Geometry: see drawing. Coordinates: mm, zero at the bounding-box minimum. Round coordinates to 2 decimals unless told otherwise and drop trailing zeros. Order: outer loops, then holes, each group sorted by start corner. A loop starts at its lowest first (then second) coordinate and runs counter-clockwise, first axis right, second up. Notation, with made-up numbers: (30, 17) -> (82, 17) arc R22 ccw to (82, 31) -> close; hole circle Ø7 at (68.5, 54.25). An arc over 180 degrees is marked (long way). Answer as CSV lines item,"result". Start each with the question number.
(1) Section query B-B (y = 3). Output: boundary loops of the cut face in (x, z), plus the area to 3 significant figures.
(2) Section query C-C (x = 1.1). Output: boundary loops of the cut face in (y, z).
(3) Section query A-A (z = 3). Output: boundary loops of the cut face in (x, y), plus the area to 3 significant figures.
(4) Line query: line 1 along Z through (x, y) = (0.6, 55); line 2 along Y through (x, z) = (1.4, 2.8); line 3 along Y through (x, z) = (0.7, 2.35). Output: solid intervals per line, ascending. Write a range as from..to.
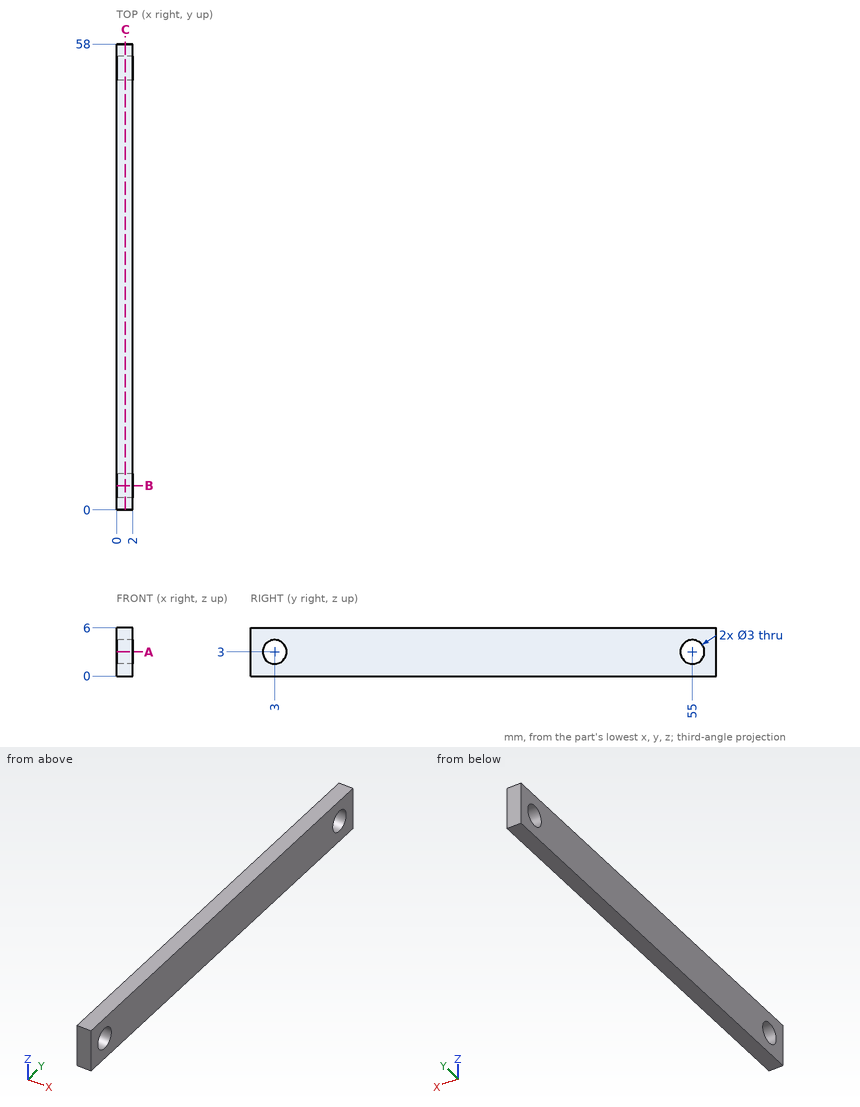
Answer block:
1,outline,"(0, 0) -> (2, 0) -> (2, 1.5) -> (0, 1.5) -> close; (0, 4.5) -> (2, 4.5) -> (2, 6) -> (0, 6) -> close"
1,area,"6.00 mm2"
2,outline,"(0, 0) -> (58, 0) -> (58, 6) -> (0, 6) -> close; hole circle Ø3 at (3, 3); hole circle Ø3 at (55, 3)"
3,outline,"(0, 0) -> (2, 0) -> (2, 1.5) -> (0, 1.5) -> close; (0, 4.5) -> (2, 4.5) -> (2, 53.5) -> (0, 53.5) -> close; (0, 56.5) -> (2, 56.5) -> (2, 58) -> (0, 58) -> close"
3,area,"104 mm2"
4,line 1,"0..1.5, 4.5..6"
4,line 2,"0..1.51, 4.49..53.51, 56.49..58"
4,line 3,"0..1.65, 4.35..53.65, 56.35..58"
